Verification items for the finished model (mm, model axes). Face numbers are marked on the shaded views. A direction names the side the tool comes from. Give positions to 0.01 mm unless a question says otherwise; leave off trailing zeros. Order: outer loops, then holes, each group sorted by start corner. A loop starts at its lowest first (then second) coordinate and runs counter-clockwise, first axis right, second up. Notation, with made-up numbers: (65.5, -8.5) - (122.5, -8.5) arc R21 ccw to (122.5, -0.5) - close; hole circle Ø3 at (-35, 32). An arc over 180 degrees is marked (long way). Answer as a JSON object with one key per item and string values. Group by question number.
(1) Section check C-C (x = -17). Record the boundary of the cut face in (y, z).
(2) Section check A-A (y = -23). Record the boundary of the cut face in (x, z).
(3) Section check B-B (x = 15.5). Record the boundary of the cut face in (y, z).
(4) Thickness scan on line 1 (Y direction, x = 8, z = 3.25); line 2 (Z direction, x = -32, y = -12.5); line 3 (Y direction, x = 15, z = 9). Record the ranges inside material, lowest first.
(5) Access from +Z, -Z, +X, -X, +Y, -Y to the whole of each face (thin tool, end or side, straight path). Record for the marked faces 1 and 2.
(6) Depth check by flat-ended pin: pin 1 Ø5 at (x, y) = (23.37, 56.47) entering from -Z; pin 2 Ø3.5 at (x, y) = (-23.28, -87.45) entering from +Z; pin 3 Ø6.5 at (x, y) = (-24.5, -88) entering from +Z; pin 4 Ø5 at (x, y) = (-41, 0) entering from +Z. Enter the tip coordinate at first touch or a pass-through.
(7) Mould release check, pull along X, two halves, no side actions. Record for the marked faces 3, 4, 5 and 6: +X half, -X half, draft (parallel to the pull), parting line (faces both ways), or undercut.
(8) Section check D-D (y = -64). Record the boundary of the cut face in (x, z), then the cut area to 3 significant figures.
```python
from build123d import *

# Parameters (mm, degrees)
EXTRUDE1_DEPTH     = 15
CHAMFER1_SIZE      = 15
CHAMFER1_SIZE2     = 8.660254038
SHELL1_T           = -2
EXTRUDE2_REACH     = 119.048
SKETCH2_R          = 4
SKETCH2_R_2        = 1.6
SKETCH3_R          = 3
CUT_EXTRUDE1_DEPTH = 15
SKETCH5_R          = 1.6
CUT_EXTRUDE2_DEPTH = 20


with BuildPart() as part:
    # Sketch1 → Extrude1 (new body)
    with BuildSketch(Plane.XY):
        Polygon((-24.967783135, 105), (-49.5, 29), (-49.5, -29), (-24.967783135, -105), (24.967783135, -105), (33.5, -29), (33.5, 29), (24.967783135, 105), align=None)
    extrude(amount=EXTRUDE1_DEPTH)

    # Chamfer1
    chamfer1_edges = [part.edges().sort_by_distance(p)[0] for p in [
        (-49.5, 0, 15),
        (-37.233891568, -67, 15),
        (0, -105, 15),
        (29.233891568, -67, 15),
        (33.5, 0, 15),
        (29.233891568, 67, 15),
        (0, 105, 15),
        (-37.233891568, 67, 15),
    ]]
    chamfer1_side = [part.faces().sort_by_distance(p)[0] for p in [
        (-5.515477183, 0, 15),
    ]]
    chamfer(chamfer1_edges, length=CHAMFER1_SIZE, length2=CHAMFER1_SIZE2, reference=chamfer1_side[0])

    # Shell1
    shell1_openings = [part.faces().sort_by_distance(p)[0] for p in [
        (-5.515477183, 0, 0),
    ]]
    offset(amount=SHELL1_T, openings=shell1_openings, kind=Kind.INTERSECTION)

    # Sketch2 → Extrude2 (add, up to next)
    with BuildSketch(Plane(origin=(0, 0, 0), x_dir=(-1, 0, 0), z_dir=(0, 0, -1)), mode=Mode.PRIVATE) as extrude2_sk1:
        with Locations((23.2777341, 87.448162672)):
            Circle(SKETCH2_R)
        with Locations((23.2777341, 87.448162672)):
            Circle(SKETCH2_R_2, mode=Mode.SUBTRACT)
    extrude2_tool1 = extrude(extrude2_sk1.sketch, amount=-EXTRUDE2_REACH, mode=Mode.PRIVATE) - part.part
    # Sketch2 → Extrude2 (add, up to next)
    with BuildSketch(Plane(origin=(0, 0, 0), x_dir=(-1, 0, 0), z_dir=(0, 0, -1)), mode=Mode.PRIVATE) as extrude2_sk2:
        with Locations((-23.372488986, 56.466339116)):
            Circle(SKETCH2_R)
        with Locations((-23.372488986, 56.466339116)):
            Circle(SKETCH2_R_2, mode=Mode.SUBTRACT)
    extrude2_tool2 = extrude(extrude2_sk2.sketch, amount=-EXTRUDE2_REACH, mode=Mode.PRIVATE) - part.part
    # Sketch2 → Extrude2 (add, up to next)
    with BuildSketch(Plane(origin=(0, 0, 0), x_dir=(-1, 0, 0), z_dir=(0, 0, -1)), mode=Mode.PRIVATE) as extrude2_sk3:
        with Locations((42.5, 0)):
            Circle(SKETCH2_R)
        with Locations((42.5, 0)):
            Circle(SKETCH2_R_2, mode=Mode.SUBTRACT)
    extrude2_tool3 = extrude(extrude2_sk3.sketch, amount=-EXTRUDE2_REACH, mode=Mode.PRIVATE) - part.part
    # Sketch2 → Extrude2 (add, up to next)
    with BuildSketch(Plane(origin=(0, 0, 0), x_dir=(-1, 0, 0), z_dir=(0, 0, -1)), mode=Mode.PRIVATE) as extrude2_sk4:
        with Locations((-23.372488986, -56.466339116)):
            Circle(SKETCH2_R)
        with Locations((-23.372488986, -56.466339116)):
            Circle(SKETCH2_R_2, mode=Mode.SUBTRACT)
    extrude2_tool4 = extrude(extrude2_sk4.sketch, amount=-EXTRUDE2_REACH, mode=Mode.PRIVATE) - part.part
    # Sketch2 → Extrude2 (add, up to next)
    with BuildSketch(Plane(origin=(0, 0, 0), x_dir=(-1, 0, 0), z_dir=(0, 0, -1)), mode=Mode.PRIVATE) as extrude2_sk5:
        with Locations((23.2777341, -87.448162672)):
            Circle(SKETCH2_R)
        with Locations((23.2777341, -87.448162672)):
            Circle(SKETCH2_R_2, mode=Mode.SUBTRACT)
    extrude2_tool5 = extrude(extrude2_sk5.sketch, amount=-EXTRUDE2_REACH, mode=Mode.PRIVATE) - part.part
    add(extrude2_tool1.solids().sort_by_distance((-19.390871, 87.448163, 0))[0])
    add(extrude2_tool2.solids().sort_by_distance((27.259352, 56.466339, 0))[0])
    add(extrude2_tool3.solids().sort_by_distance((-38.613137, 0, 0))[0])
    add(extrude2_tool4.solids().sort_by_distance((27.259352, -56.466339, 0))[0])
    add(extrude2_tool5.solids().sort_by_distance((-19.390871, -87.448163, 0))[0])

    # Sketch3 → Cut-Extrude1 (cut)
    with BuildSketch(Plane(origin=(0, 0, 3), x_dir=(-1, 0, 0), z_dir=(0, 0, -1))):
        with Locations((23.2777341, 87.448162672)):
            Circle(SKETCH3_R)
        with Locations((-23.372488986, 56.466339116)):
            Circle(SKETCH3_R)
        with Locations((-23.372488986, -56.466339116)):
            Circle(SKETCH3_R)
        with Locations((23.2777341, -87.448162672)):
            Circle(SKETCH3_R)
        with Locations((42.5, 0)):
            Circle(SKETCH3_R)
    extrude(amount=-CUT_EXTRUDE1_DEPTH, mode=Mode.SUBTRACT)

    # Sketch5 → Cut-Extrude2 (cut)
    with BuildSketch(Plane.XY.offset(19)):
        with Locations((-10.967783135, 55.6)):
            Circle(SKETCH5_R)
        with Locations((7.032216865, 55.6)):
            Circle(SKETCH5_R)
        with Locations((7.032216865, -55.6)):
            Circle(SKETCH5_R)
        with Locations((-10.967783135, -55.6)):
            Circle(SKETCH5_R)
    extrude(amount=-CUT_EXTRUDE2_DEPTH, mode=Mode.SUBTRACT)


solid = part.part
```
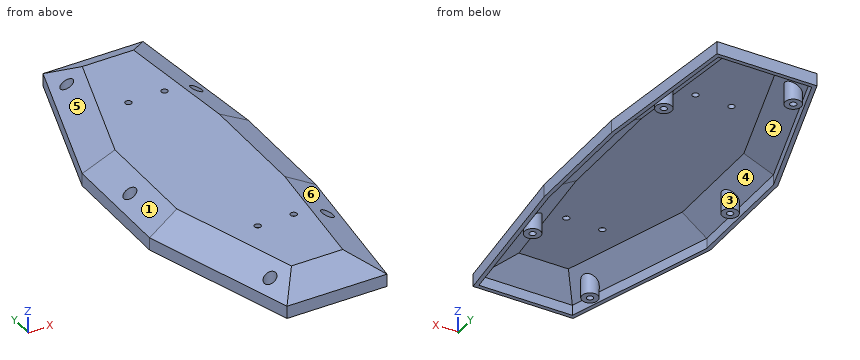
Solutions:
{
 "1": {"outline": "(-105, 0) - (-103, 0) - (-103, 5.19) - (-94.06, 10.35) - (-79.11, 13) - (79.11, 13) - (94.06, 10.35) - (103, 5.19) - (103, 0) - (105, 0) - (105, 6.34) - (94.06, 12.66) - (80.85, 15) - (-80.85, 15) - (-94.06, 12.66) - (-105, 6.34) - close"},
 "2": {"outline": "(-49.5, 0) - (-47.5, 0) - (-47.5, 5.19) - (-33.96, 13) - (17.96, 13) - (31.5, 5.19) - (31.5, 0) - (33.5, 0) - (33.5, 6.34) - (18.5, 15) - (-34.5, 15) - (-49.5, 6.34) - close"},
 "3": {"outline": "(-105, 0) - (-103, 0) - (-103, 5.19) - (-94.41, 10.14) - (-50.08, 13) - (50.08, 13) - (94.41, 10.14) - (103, 5.19) - (103, 0) - (105, 0) - (105, 6.34) - (94.41, 12.45) - (54.88, 15) - (-54.88, 15) - (-94.41, 12.45) - (-105, 6.34) - close"},
 "4": {"line 1": "y = -105 to -103, 103 to 105", "line 2": "z = 13 to 15", "line 3": "y = -100.39 to -96.39, 96.39 to 100.39"},
 "5": {"face 1": "+Z, -X, +Y, -Y", "face 2": "-Z"},
 "6": {"pin 1": "stops at z = 0", "pin 2": "stops at z = 3", "pin 3": "stops at z = 10.52", "pin 4": "stops at z = 12.69"},
 "7": {"face 3": "undercut", "face 4": "undercut", "face 5": "-X half", "face 6": "+X half"},
 "8": {"outline": "(-38.2, 0) - (-36.1, 0) - (-36.1, 5.19) - (-21.88, 13) - (13.94, 13) - (27.56, 5.19) - (27.56, 0) - (29.57, 0) - (29.57, 6.34) - (14.48, 15) - (-22.44, 15) - (-38.2, 6.34) - close", "area": "164 mm2"}
}
